Can you work these out from the model? Positions are in its coordinate system, mm. A direction names the side the tool comes from. Round coordinates to 2 decimals unless told otherwise and drop trailing zeros. Loops run counter-clockwise (first coordinate to the right, second up) from the corner with the lowest first, then second, coordinate; pieces in that order, holes last. Notation, with made-up numbers: M 41,41 L 51,41 A22 cw 51,61 Z; hole C -17,34.25 d8. An arc over 180 degrees is marked long. Return JSON: item names as keys, results as strings.
```python
from build123d import *

# Parameters (mm, degrees)
BOSS_EXTRUDE1_DEPTH      = 48.26
BOSS_EXTRUDE1_DEPTH_BACK = 48.26
SKETCH3_R                = 3.96875
CHAMFER1_SIZE            = 0.555625
CUT_EXTRUDE1_START       = -1.905
SKETCH4_R                = 18.115105144
SKETCH4_R_2              = 3.8
CUT_EXTRUDE1_DEPTH       = 0.899999978


with BuildPart() as part:
    # Sketch3 → Boss-Extrude1 (new, two sides: drawn at the far end of the back side and taken through both)
    with BuildSketch(Plane.XY.offset(-BOSS_EXTRUDE1_DEPTH_BACK)):
        with Locations(Location((0, 0, 0), (0, 0, 180))):
            Circle(SKETCH3_R)
    extrude(amount=BOSS_EXTRUDE1_DEPTH + BOSS_EXTRUDE1_DEPTH_BACK)

    # Chamfer1
    chamfer1_edges = [part.edges().sort_by_distance(p)[0] for p in [
        (3.96875, 0, -48.26),
        (3.96875, 0, 48.26),
    ]]
    chamfer(chamfer1_edges, length=CHAMFER1_SIZE)

    # Sketch4 → Cut-Extrude1 (cut)
    with BuildSketch(Plane.XY.offset(48.26).offset(CUT_EXTRUDE1_START)):
        Circle(SKETCH4_R)
        Circle(SKETCH4_R_2, mode=Mode.SUBTRACT)
    cut_extrude1 = extrude(amount=-CUT_EXTRUDE1_DEPTH, mode=Mode.SUBTRACT)

    # Mirror1: Cut-Extrude1 across plane
    add(cut_extrude1.mirror(Plane.XY), mode=Mode.SUBTRACT)


solid = part.part
```
Q1. If I drill on line 1 along X through (y, z) = (0.25, 3.5); line 2 along Y through (x, z) = (-0.75, -27.5), over which ranges is the centre line in solid material (lowest first)?
Results:
{"line 1": "x = -3.96 to 3.96", "line 2": "y = -3.9 to 3.9"}
Q2. On a 3-axis mill with a long thin cutter (end or side, diameter ignored), from which of +Z, -Z, +X, -X, +Y, -Y can I reach the whole of each face in a straight line? I mean faces 4 (the cylindrical face through (-3.796, 0.167, -45.911)), 5 (the flat face through (0, 0, -48.26)). Say none if no direction works.
Results:
{"face 4": "none", "face 5": "-Z, +X, -X, +Y, -Y"}
Q3. I'm going to push flat-ended pins straight in: pin 1 Ø3 at (y, z) = (2.5, -22) entering from +X; pin 2 Ø2 at (y, z) = (2, -15.5) entering from -X. Where does each tip first touch, or does it pass through?
Results:
{"pin 1": "stops at x = 3.84", "pin 2": "stops at x = -3.84"}
Q4. Suppose I cut it at A-A, the plane z = 30. Please give me the cut outline in (x, y), plus the area to 3 significant figures.
Results:
{"outline": "C 0,0 d7.94", "area": "49.5 mm2"}
Q5. Thinking about a two-plate mould opening in Z: for faces 1 (the cylindrical face through (-3.796, 0.167, 45.911)), 2 (the flat face through (0, 0, 48.26)), 3 (the cylindrical face through (0.86, 3.874, -0.636)), which applies, pulls with the +Z half, pulls with the -Z half, needs draft (parallel to the pull), parting line crosses it, or undercut?
Results:
{"face 1": "undercut", "face 2": "pulls with the +Z half", "face 3": "needs draft"}
